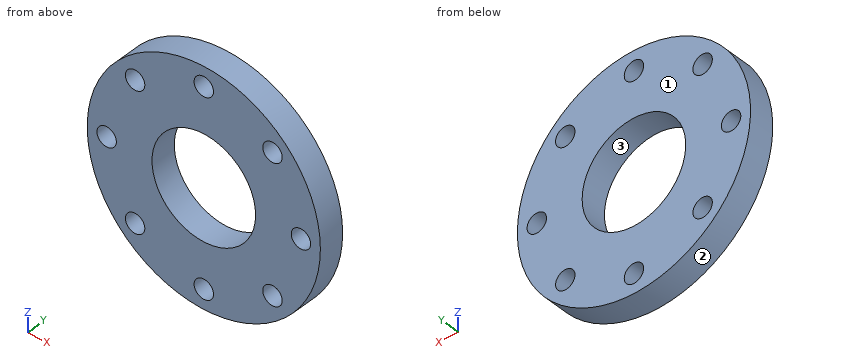
from build123d import *

# Parameters (mm, degrees)
F0_R     = 114.3
F0_R_2   = 50.8
F1_DEPTH = 25.4
F2_R     = 9.525
F3_DEPTH = 25.4


with BuildPart() as f1:
    # F0 (on Front) → F1 (new body)
    with BuildSketch(Plane.XZ):
        Circle(F0_R)
        Circle(F0_R_2, mode=Mode.SUBTRACT)
    extrude(amount=F1_DEPTH)

    # F2 (on face) → F3 (cut, through all)
    with BuildSketch(Plane.XZ.offset(25.4)):
        with Locations((0, 95.25)):
            Circle(F2_R)
        with Locations((-67.351921, 67.351921)):
            Circle(F2_R)
        with Locations((-95.25, 0)):
            Circle(F2_R)
        with Locations((-67.351921, -67.351921)):
            Circle(F2_R)
        with Locations((0, -95.25)):
            Circle(F2_R)
        with Locations((67.351921, -67.351921)):
            Circle(F2_R)
        with Locations((95.25, 0)):
            Circle(F2_R)
        with Locations((67.351921, 67.351921)):
            Circle(F2_R)
    extrude(amount=-F3_DEPTH, mode=Mode.SUBTRACT)


solid = f1.part
Could you check a few things on this model? Use its own coordinates, in mm. Face numbers are marked on the shaded views. Coordinates: 2 decimals unless noted, no trailing zeros. Order: outer loops, then holes, each group sorted by start corner. A loop starts at its lowest first (then second) coordinate and runs counter-clockwise, first axis right, second up. Notation, with made-up numbers: (-7.5, 31) -> (50.5, 31) arc R35 ccw to (50.5, 69) -> close; hole circle Ø7 at (83, 34.25). An arc over 180 degrees is marked (long way). One line per item, written item: value. Start each with the question number.
1) If I drill on L1, parallel to Z at x = 0, y = -13.25 (3 decimals); L2, parallel to Z at x = -2.5, y = -3.5; L3, parallel to X at y = -16.5, z = 3.5, over which ranges is the centre line in solid material (lowest first)? Write a range as [from, to].
2) We'd pull the mould along X, two halves only. Please class the marked faces 1, 2 and 3: +X half, -X half, draft (parallel to the pull), parting line (faces both ways), or undercut.
3) I'm going to push flat-ended pins straight in: pin 1 (6 mm diameter, centred on y = -12, z = 13, fed in from +X); pin 2 (15 mm diameter, centred on x = -67.35, z = -67.35, fed in from +Y); pin 3 (3 mm diameter, centred on x = -9, y = -15.5, fed in from +Z); pin 4 (12 mm diameter, centred on y = -20, z = 36, fed in from -X). Where does each tip first touch, or does it pass through?
4) Imagine slicing it at C-C on z = 60.5. List the corners of the cut face in (x, y) for me.
5) Imagine slicing it at B-B on x = 89.5. List the corners of the cut face in (y, z) for me, plus the area to 3 significant figures.
6) Imagine slicing it at A-A on z = 0. List the corners of the cut face in (x, y) for me (3 decimals).
7) Imagine slicing it at D-D on y = -16.5. Count the separate pieces of the cut face and the enclosed holes in it, plus the area to 3 significant figures.
Answer list:
1. L1: z = [-114.3, -104.775], [-85.725, -50.8], [50.8, 85.725], [104.775, 114.3]
1. L2: z = [-114.27, -104.44], [-86.06, -50.74], [50.74, 86.06], [104.44, 114.27]
1. L3: x = [-114.25, -104.11], [-86.39, -50.68], [50.68, 86.39], [104.11, 114.25]
2. face 1: draft
2. face 2: parting line
2. face 3: undercut
3. pin 1: stops at x = 113.86
3. pin 2: passes through
3. pin 3: stops at z = 114.05
3. pin 4: stops at x = -110.29
4. outline: (-96.98, -25.4) -> (-73.97, -25.4) -> (-73.97, 0) -> (-96.98, 0) -> close; (-60.74, -25.4) -> (60.74, -25.4) -> (60.74, 0) -> (-60.74, 0) -> close; (73.97, -25.4) -> (96.98, -25.4) -> (96.98, 0) -> (73.97, 0) -> close
5. outline: (-25.4, -71.09) -> (0, -71.09) -> (0, -7.59) -> (-25.4, -7.59) -> close; (-25.4, 7.59) -> (0, 7.59) -> (0, 71.09) -> (-25.4, 71.09) -> close
5. area: 3,230 mm2
6. outline: (-114.3, -25.4) -> (-104.775, -25.4) -> (-104.775, 0) -> (-114.3, 0) -> close; (-85.725, -25.4) -> (-50.8, -25.4) -> (-50.8, 0) -> (-85.725, 0) -> close; (50.8, -25.4) -> (85.725, -25.4) -> (85.725, 0) -> (50.8, 0) -> close; (104.775, -25.4) -> (114.3, -25.4) -> (114.3, 0) -> (104.775, 0) -> close
7. separate pieces: 1
7. enclosed holes: 9
7. area: 30,700 mm2
